from build123d import *

# Parameters (mm, degrees)
BOSS_EXTRUDE1_DEPTH = 1.3
SKETCH2_R           = 1.27
CUT_EXTRUDE2_DEPTH  = 43.086324906


with BuildPart() as part:
    # Sketch1 → Boss-Extrude1 (new body)
    with BuildSketch(Plane(origin=(0, 0, 0), x_dir=(1, 0, 0), z_dir=(0, 1, 0))):
        Polygon((21.57246336, -21.977580043), (29.819374311, 7.693511271), (8.246910951, 29.671091314), (-21.57246336, 21.977580043), (-29.819374311, -7.693511271), (-8.246910951, -29.671091314), align=None)
    extrude(amount=BOSS_EXTRUDE1_DEPTH)

    # Sketch2 → Cut-Extrude2 (cut, through all)
    with BuildSketch(Plane(origin=(0, 0, 0), x_dir=(1, 0, 0), z_dir=(0, 1, 0))):
        with Locations(Location((6.801937511, 24.472303653, 0), (0, 0, 270))):
            Circle(SKETCH2_R)
        with Locations(Location((24.594605408, 6.345501147, 0), (0, 0, 270))):
            Circle(SKETCH2_R)
        with Locations(Location((17.792667898, -18.126802506, 0), (0, 0, 270))):
            Circle(SKETCH2_R)
        with Locations(Location((-6.801937511, -24.472303653, 0), (0, 0, 270))):
            Circle(SKETCH2_R)
        with Locations(Location((-24.594605408, -6.345501147, 0), (0, 0, 270))):
            Circle(SKETCH2_R)
        with Locations(Location((-17.792667898, 18.126802506, 0), (0, 0, 270))):
            Circle(SKETCH2_R)
    extrude(amount=CUT_EXTRUDE2_DEPTH, mode=Mode.SUBTRACT)


solid = part.part
For this review, take the finished solid that the model builds, in its own axes (mm). Round coordinates to 2 decimals unless told otherwise and drop trailing zeros. Write each loop counter-clockwise with the first axis right and the second up, starting at its lowest first coordinate (ties: lowest second). Pieces come first, ordered by that corner, then holes. Notation, with made-up numbers: (-5.75, 83.5) - (6.25, 83.5) arc R14 cw to (6.25, 106.5) - close; hole circle Ø10 at (-5.5, 29). An arc over 180 degrees is marked (long way). Write item = value, one per line. Start each with the question number.
1. Consider section A-A on y = 0.85. State the section outline as (x, z) points.
2. Consider section D-D on z = -2. State the section outline as (x, y) points.
3. Wall thickness on L1, parallel to X at y = 0.6, z = 19; L2, parallel to X at y = 0.8, z = -6.5; L3, parallel to Z at x = 12, y = 0.55: over which ranges is each line inside the solid? List them lowest first.
4. Draft analysis for pull direction X (two halves, no side actions). For faces 1 (the face through (25.64, 0.64, 7.35)), 2 (the face through (-25.64, 0.64, -7.35)), 3 (the face through (-7.288, 0.641, 25.645)), state which applies: released by +X, released by -X, zero draft, split by the parting line, or undercut.
5. Consider section B-B on z = 24.5. State the section outline as (x, y) points, plus the area to 3 significant figures.
6. Consider section C-C on x = -13.5. State the section outline as (y, z) points.
7. For pin 1 Ø1.5 at (x, z) = (17.79, 18.13) entering from +Y, flat-tipped, find the tip position at first contact; note if it passes through.
Evaluation:
q1.outline = (-29.82, 7.69) - (-21.57, -21.98) - (8.25, -29.67) - (29.82, -7.69) - (21.57, 21.98) - (-8.25, 29.67) - close; hole circle Ø2.54 at (-24.59, 6.35); hole circle Ø2.54 at (-17.79, -18.13); hole circle Ø2.54 at (-6.8, 24.47); hole circle Ø2.54 at (6.8, -24.47); hole circle Ø2.54 at (17.79, 18.13); hole circle Ø2.54 at (24.59, -6.35)
q2.outline = (-27.13, 0) - (28.24, 0) - (28.24, 1.3) - (-27.13, 1.3) - close
q3.L1 = -18.72 to 16.87, 18.71 to 22.4
q3.L2 = -25.87 to 23.33, 25.86 to 29.49
q3.L3 = -25.85 to 24.45
q4.face_1 = released by +X
q4.face_2 = released by -X
q4.face_3 = undercut
q5.outline = (-13.32, 0) - (-8.07, 0) - (-8.07, 1.3) - (-13.32, 1.3) - close; (-5.53, 0) - (11.8, 0) - (11.8, 1.3) - (-5.53, 1.3) - close
q5.area = 29.4 mm2
q6.outline = (0, -24.06) - (1.3, -24.06) - (1.3, 24.32) - (0, 24.32) - close
q7.pin_1 = through
